Print and shaded views of the part. All mm, measured from the part's lowest x, y and z. A direction names the side the tool comes from. Round coordinates to 2 decimals unless told otherwise and drop trailing zeros. Loops run counter-clockwise (first coordinate to the right, second up) from the corner with the lowest first, then second, coordinate; pieces in that order, holes last. Notation, with made-up numbers: (37.5, 86.5) - (78.5, 86.5) arc R17 cw to (78.5, 110.5) - close; hole circle Ø8 at (-21, -5.5). An arc over 180 degrees is marked (long way). Put each result on its own line as item: value. Start each with the question number.
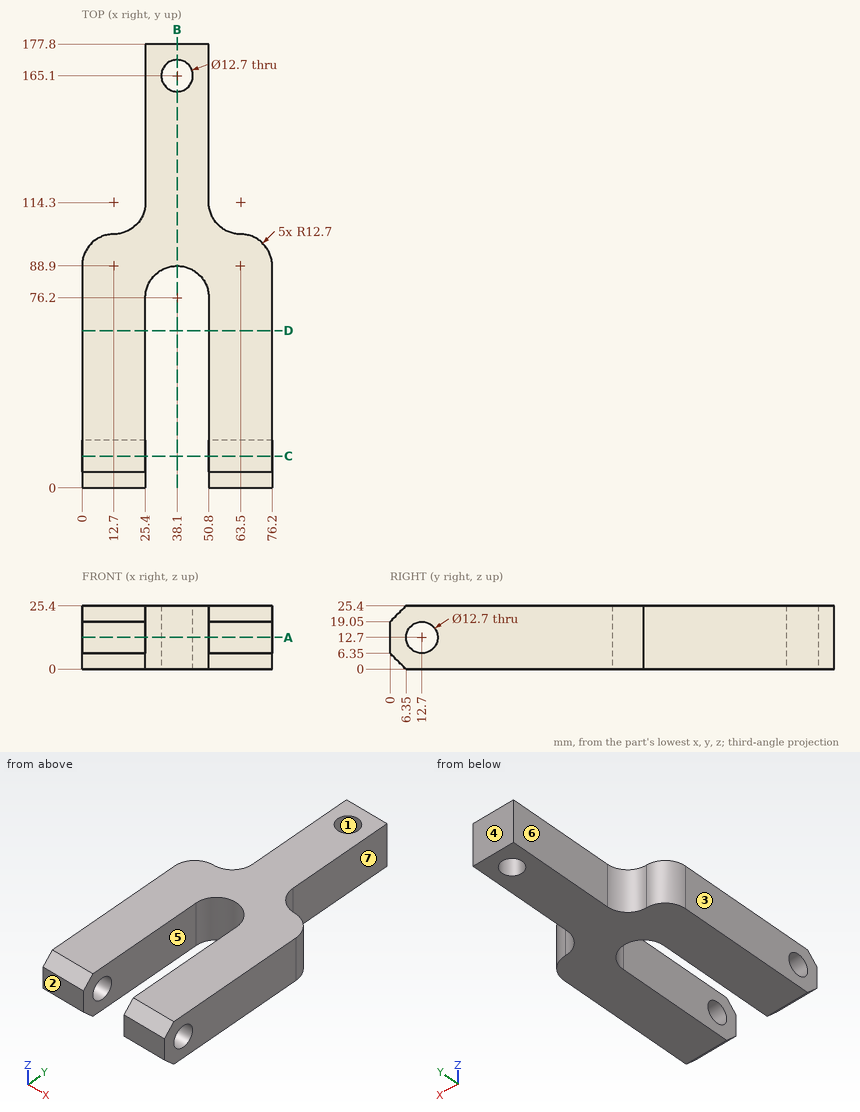
Item 1: Which spindle directions (+Z, -Z, +X, -X, +Y, -Y) get a long thin tool onto all of the face, cutting with end or side? Do the marked faces 5, 6 and 7. Say none if no direction does.
Item 2: Slice it at D-D (y = 63). Give the cut face in (x, z), plus the area to 3 significant figures.
Item 3: Two-plate mould, pull along Y, no slides. Class the marked faces 1, 2, 3 and 4: pulls with the +Y half, pulls with the -Y half, needs draft (parallel to the pull), parting line crosses it, or undercut.
Item 4: Drill centre lines: probe 1 along X at (y, z) = (77, 14.25); probe 2 along Y at (x, z) = (38.1, 9); probe 3 along X at (y, z) = (136, 10.5). Where is each one in solid material? Low to high. Write a range as [from, to].
Item 5: Slice it at A-A (z = 12.7). Give the cut face in (x, y), plus the area to 3 significant figures.
Item 6: Slice it at C-C (y = 12.7). Give the cut face in (x, z), plus the area to 3 significant figures.
Item 7: Drop flat-ended pins along their axis: pin 1 Ø1 at (x, z) = (23, 10) entering from +Y; pin 2 Ø12.5 at (y, z) = (136.5, 13) entering from -X; pin 3 Ø1 at (x, z) = (49, 22) entering from -Y. Give the stop position or say it passes through.
Item 8: Slice it at B-B (x = 38.1). Give the cut face in (y, z), plus the area to 3 significant figures.
Computed values:
1. face 5: +Z, -Z, -Y
1. face 6: +Z, -Z, -X, +Y
1. face 7: +Z, -Z, +X, +Y
2. outline: (0, 0) - (25.4, 0) - (25.4, 25.4) - (0, 25.4) - close; (50.8, 0) - (76.2, 0) - (76.2, 25.4) - (50.8, 25.4) - close
2. area: 1,290 mm^2
3. face 1: undercut
3. face 2: pulls with the -Y half
3. face 3: needs draft
3. face 4: pulls with the +Y half
4. probe 1: x = [0, 25.43], [50.77, 76.2]
4. probe 2: y = [88.9, 158.75], [171.45, 177.8]
4. probe 3: x = [25.4, 50.8]
5. outline: (0, 0) - (25.4, 0) - (25.4, 6.35) - (0, 6.35) - close; (0, 19.05) - (25.4, 19.05) - (25.4, 76.2) arc R12.7 cw to (50.8, 76.2) - (50.8, 19.05) - (76.2, 19.05) - (76.2, 88.9) arc R12.7 ccw to (63.5, 101.6) arc R12.7 cw to (50.8, 114.3) - (50.8, 177.8) - (25.4, 177.8) - (25.4, 114.3) arc R12.7 cw to (12.7, 101.6) arc R12.7 ccw to (0, 88.9) - close; (50.8, 0) - (76.2, 0) - (76.2, 6.35) - (50.8, 6.35) - close; hole circle Ø12.7 at (38.1, 165.1)
5. area: 6,720 mm^2
6. outline: (0, 0) - (25.4, 0) - (25.4, 6.35) - (0, 6.35) - close; (0, 19.05) - (25.4, 19.05) - (25.4, 25.4) - (0, 25.4) - close; (50.8, 0) - (76.2, 0) - (76.2, 6.35) - (50.8, 6.35) - close; (50.8, 19.05) - (76.2, 19.05) - (76.2, 25.4) - (50.8, 25.4) - close
6. area: 645 mm^2
7. pin 1: stops at y = 107.62
7. pin 2: stops at x = 25.4
7. pin 3: stops at y = 81.8
8. outline: (88.9, 0) - (158.75, 0) - (158.75, 25.4) - (88.9, 25.4) - close; (171.45, 0) - (177.8, 0) - (177.8, 25.4) - (171.45, 25.4) - close
8. area: 1,940 mm^2
